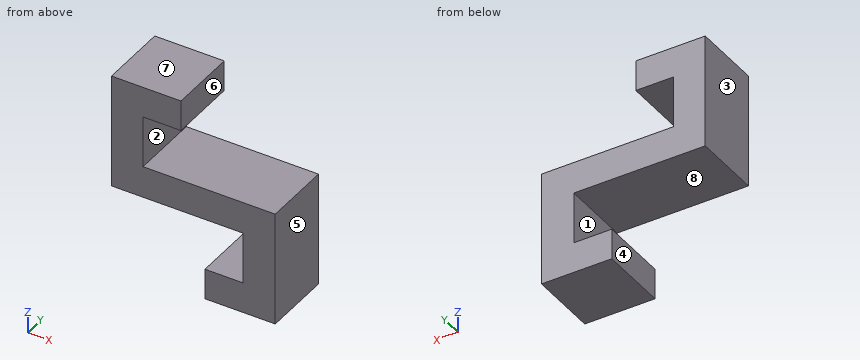
Autodesk Inventor part; units mm, degrees
ref_plane "YZ Plane" through (0, 0, 0) normal (1, 0, 0) x (0, 1, 0)
ref_plane "XZ Plane" through (0, 0, 0) normal (0, 1, 0) x (-1, 0, 0)
ref_plane "XY Plane" through (0, 0, 0) normal (0, 0, 1) x (1, 0, 0)
sketch "Skizze1" plane through (0, 0, 0) normal (0, 1, 0) x (-1, 0, 0)
  line L0 (-10.1354, -12.1625) -> (-1.4354, -12.1625)
  line L1 (10.1354, -1.9625) -> (10.1354, 12.1625)
  line L2 (10.1354, 12.1625) -> (1.5354, 12.1625)
  line L3 (-10.1354, 1.9625) -> (-10.1354, -12.1625)
  line L4 (-10.1354, -12.1625) -> (10.1354, 12.1625) construction
  line L5 (10, -12) -> (-10, 12) construction
  line L6 (1.5354, 12.1625) -> (1.5354, 8.3625)
  line L7 (1.5354, 8.3625) -> (6.2354, 8.3625)
  line L8 (6.2354, 8.3625) -> (6.2354, 1.9625)
  line L9 (6.2354, 1.9625) -> (-10.1354, 1.9625)
  line L10 (-1.4354, -12.1625) -> (-1.4354, -8.3625)
  line L11 (-1.4354, -8.3625) -> (-6.1354, -8.3625)
  line L12 (-6.1354, -8.3625) -> (-6.1354, -1.9625)
  line L13 (-6.1354, -1.9625) -> (10.1354, -1.9625)
  point P0 (0, 0)
  point P1 (1.5354, 10.2625)
  point P2 (6.2354, 5.1625)
  point P3 (-1.4354, -10.2625)
  dimension "d12" = 6.4
  dimension "d13" = 3.8
  dimension "d14" = 6.4
  dimension "d15" = 3.925
  dimension "d16" = 3.9
  dimension "d17" = 3.8
  dimension "d18" = 4.7
  dimension "d19" = 4.7
extrude "Extrusion1" add sketch "Skizze1" along normal blind 8.6
properties part number "Haken für Bioprinter 4x9mm 001"
Here's how the part is built. I have some questions about the finished solid (model axes, mm). Face numbers are marked on the shaded views. A direction names the side the tool comes from. Round coordinates to 2 decimals unless told otherwise and drop trailing zeros. Loops run counter-clockwise (first coordinate to the right, second up) from the corner with the lowest first, then second, coordinate; pieces in that order, holes last. Notation, with made-up numbers: (11, -23.5) -> (26, -23.5) arc R11 cw to (26, -13.5) -> close; hole circle Ø3 at (-26, -11.75). An arc over 180 degrees is marked (long way). Answer as CSV lines item,"result". Start each with the question number.
1. For the marked faces 1, 2, 3, 4 and 5, which set-ups out of +Z, -Z, +X, -X, +Y, -Y let a thin tool reach every point of the face, with its end or its side?
2. I need wall thicknesses on probe 1 along Z at (x, y) = (-1.75, 7.75); probe 2 along Z at (x, y) = (2, 2); probe 3 along Z at (x, y) = (6.75, 3). Which ranges of each line are inside material? Lowest first, please. Write a range as from..to.
3. Imagine slicing it at C-C on z = 7.5. Write out the boundary of the cut face in (x, y).
4. Imagine slicing it at A-A on x = 4. Write out the boundary of the cut face in (y, z), plus the area to 3 significant figures.
5. Imagine slicing it at B-B on y = 4.5. Write out the boundary of the cut face in (x, z), plus the area to 3 significant figures.
6. If we mould it in two halves opening along Z, with no side actions, what happens to the marked faces 6, 7 and 8? For each: pulls with the +Z half, pulls with the -Z half, needs draft (parallel to the pull), parting line crosses it, or undercut.
7. Imagine slicing it at D-D on z = -5. Write out the boundary of the cut face in (x, y), plus the area to 3 significant figures.
8. I'm going to push flat-ended pins straight in: P1, Ø1.9, axis at y = 3.5, z = -10.5, coming from the -X side; P2, Ø4, axis at x = -2.5, z = -8.5, coming from the -Y side; P3, Ø4.5, axis at x = 1, y = 4, coming from the +Z side; P4, Ø2.5, axis at x = -4.5, y = 5, coming from the -Z side. Where does each tip first touch, or does it pass through?
Solution:
1,face 1,"-X, +Y, -Y"
1,face 2,"+X, +Y, -Y"
1,face 3,"+Z, -Z, -X, +Y, -Y"
1,face 4,"-Z, -X, +Y, -Y"
1,face 5,"+Z, -Z, +X, +Y, -Y"
2,probe 1,"-1.96..1.96, 8.36..12.16"
2,probe 2,"-12.16..-8.36, -1.96..1.96"
2,probe 3,"-12.16..1.96"
3,outline,"(-10.14, 0) -> (-6.24, 0) -> (-6.24, 8.6) -> (-10.14, 8.6) -> close"
4,outline,"(0, -12.16) -> (8.6, -12.16) -> (8.6, -8.36) -> (0, -8.36) -> close; (0, -1.96) -> (8.6, -1.96) -> (8.6, 1.96) -> (0, 1.96) -> close"
4,area,"66.4 mm²"
5,outline,"(-10.14, -1.96) -> (6.14, -1.96) -> (6.14, -8.36) -> (1.44, -8.36) -> (1.44, -12.16) -> (10.14, -12.16) -> (10.14, 1.96) -> (-6.24, 1.96) -> (-6.24, 8.36) -> (-1.54, 8.36) -> (-1.54, 12.16) -> (-10.14, 12.16) -> close"
5,area,"196 mm²"
6,face 6,"needs draft"
6,face 7,"pulls with the +Z half"
6,face 8,"undercut"
7,outline,"(6.14, 0) -> (10.14, 0) -> (10.14, 8.6) -> (6.14, 8.6) -> close"
7,area,"34.4 mm²"
8,P1,"x = 1.44"
8,P2,"through"
8,P3,"z = 1.96"
8,P4,"z = -1.96"
